from build123d import *

# Parameters (mm, degrees)
SKETCH_1_R          = 2.15
SKETCH_1_W          = 14.4
SKETCH_1_H          = 14.4
EXTRUDE_1_DEPTH     = 6
CUT_EXTRUDE_START   = -4
CUT_EXTRUDE_1_DEPTH = 4
CHAMFER_1_SIZE      = 1
SKETCH_4_W          = 5
SKETCH_4_H          = 1
CUT_EXTRUDE_2_DEPTH = 0.4


with BuildPart() as part:
    # Эскиз1 → Бобышка-Вытянуть1 (new body)
    with BuildSketch(Plane.XY):
        with BuildLine():
            Line((17.75, 16.5), (-17.75, 16.5))
            ThreePointArc((-17.75, 16.5), (-20.401650429, 15.401650429), (-21.5, 12.75))
            Line((-21.5, 12.75), (-21.5, -12.75))
            ThreePointArc((-21.5, -12.75), (-20.401650429, -15.401650429), (-17.75, -16.5))
            Line((-17.75, -16.5), (17.75, -16.5))
            ThreePointArc((17.75, -16.5), (20.401650429, -15.401650429), (21.5, -12.75))
            Line((21.5, -12.75), (21.5, 12.75))
            ThreePointArc((21.5, 12.75), (20.401650429, 15.401650429), (17.75, 16.5))
        make_face()
        with Locations((-17.75, 12.75)):
            Circle(SKETCH_1_R, mode=Mode.SUBTRACT)
        with Locations((17.75, 12.75)):
            Circle(SKETCH_1_R, mode=Mode.SUBTRACT)
        with Locations((-17.75, -12.75)):
            Circle(SKETCH_1_R, mode=Mode.SUBTRACT)
        with Locations((17.75, -12.75)):
            Circle(SKETCH_1_R, mode=Mode.SUBTRACT)
        with Locations((-9.5, 0)):
            Rectangle(SKETCH_1_W, SKETCH_1_H, mode=Mode.SUBTRACT)
        with Locations((9.5, 0)):
            Rectangle(SKETCH_1_W, SKETCH_1_H, mode=Mode.SUBTRACT)
    extrude(amount=EXTRUDE_1_DEPTH)

    # Эскиз2 → Вырез-Вытянуть1 (cut)
    with BuildSketch(Plane.XY.offset(6).offset(CUT_EXTRUDE_START)):
        with BuildLine():
            Line((-21.5, 10.25), (-20.545084972, 10.25))
            ThreePointArc((-20.545084972, 10.25), (-19.837764528, 9.634917453), (-19, 9.214466094))
            Line((-19, 9.214466094), (-19, -9.214466094))
            ThreePointArc((-19, -9.214466094), (-19.837764528, -9.634917453), (-20.545084972, -10.25))
            Line((-20.545084972, -10.25), (-21.5, -10.25))
            Line((-21.5, -10.25), (-21.5, -12.75))
            ThreePointArc((-21.5, -12.75), (-20.401650429, -15.401650429), (-17.75, -16.5))
            Line((-17.75, -16.5), (-15.25, -16.5))
            Line((-15.25, -16.5), (-15.25, -15.545084972))
            ThreePointArc((-15.25, -15.545084972), (-14.020147597, -12.361797664), (-15.879171307, -9.5))
            Line((-15.879171307, -9.5), (15.879171307, -9.5))
            ThreePointArc((15.879171307, -9.5), (14.020147597, -12.361797664), (15.25, -15.545084972))
            Line((15.25, -15.545084972), (15.25, -16.5))
            Line((15.25, -16.5), (17.75, -16.5))
            ThreePointArc((17.75, -16.5), (20.401650429, -15.401650429), (21.5, -12.75))
            Line((21.5, -12.75), (21.5, -10.25))
            Line((21.5, -10.25), (20.545084972, -10.25))
            ThreePointArc((20.545084972, -10.25), (19.837764528, -9.634917453), (19, -9.214466094))
            Line((19, -9.214466094), (19, 9.214466094))
            ThreePointArc((19, 9.214466094), (19.837764528, 9.634917453), (20.545084972, 10.25))
            Line((20.545084972, 10.25), (21.5, 10.25))
            Line((21.5, 10.25), (21.5, 12.75))
            ThreePointArc((21.5, 12.75), (20.401650429, 15.401650429), (17.75, 16.5))
            Line((17.75, 16.5), (15.25, 16.5))
            Line((15.25, 16.5), (15.25, 15.545084972))
            ThreePointArc((15.25, 15.545084972), (14.020147597, 12.361797664), (15.879171307, 9.5))
            Line((15.879171307, 9.5), (-15.879171307, 9.5))
            ThreePointArc((-15.879171307, 9.5), (-14.020147597, 12.361797664), (-15.25, 15.545084972))
            Line((-15.25, 15.545084972), (-15.25, 16.5))
            Line((-15.25, 16.5), (-17.75, 16.5))
            ThreePointArc((-17.75, 16.5), (-20.401650429, 15.401650429), (-21.5, 12.75))
            Line((-21.5, 12.75), (-21.5, 10.25))
        make_face()
    extrude(amount=CUT_EXTRUDE_1_DEPTH, mode=Mode.SUBTRACT)

    # Фаска1
    # the kernel refuses this chamfer: 1, 0.732303349 mm, written as the material it takes off along each edge
    with BuildSketch(Plane(origin=(15.879171307, 9.5, 2), x_dir=(-0.8149940779202551, 0.5794692856009827, 0), z_dir=(0, 0, 1))) as chamfer_1_piece_1:
        with BuildLine():
            Line((0.717121745, 0), (CHAMFER_1_SIZE * 0.81499407792, CHAMFER_1_SIZE * 0.579469285601))
            Line((CHAMFER_1_SIZE * 0.81499407792, CHAMFER_1_SIZE * 0.579469285601), (0, 0))
            ThreePointArc((0, 0), (0.355196947, 0.017179972), (0.717121745, 0))
        make_face()
    extrude(amount=6.571682988, mode=Mode.SUBTRACT)
    with BuildSketch(Plane(origin=(-15.879171307, 9.5, 2), x_dir=(1, 0, 0), z_dir=(0, 0, 1))) as chamfer_1_piece_2:
        with BuildLine():
            Line((CHAMFER_1_SIZE, 0), (0.584449975, 0.415550025))
            ThreePointArc((0.584449975, 0.415550025), (0.299438674, 0.191824146), (0, 0))
            Line((0, 0), (CHAMFER_1_SIZE, 0))
        make_face()
    extrude(amount=6.571682988, mode=Mode.SUBTRACT)
    with BuildSketch(Plane(origin=(15.879171307, -9.5, 2), x_dir=(-0.8149940779202558, -0.5794692856009814, 0), z_dir=(0, 0, 1))) as chamfer_1_piece_3:
        with BuildLine():
            Line((0.717121745, 0), (CHAMFER_1_SIZE * 0.81499407792, -CHAMFER_1_SIZE * 0.579469285601))
            Line((CHAMFER_1_SIZE * 0.81499407792, -CHAMFER_1_SIZE * 0.579469285601), (0, 0))
            ThreePointArc((0, 0), (0.355196947, -0.017179972), (0.717121745, 0))
        make_face()
    extrude(amount=6.571682988, mode=Mode.SUBTRACT)
    with BuildSketch(Plane(origin=(-15.879171307, -9.5, 2), x_dir=(1, 0, 0), z_dir=(0, 0, 1))) as chamfer_1_piece_4:
        with BuildLine():
            Line((CHAMFER_1_SIZE, 0), (0.584449975, -0.415550025))
            ThreePointArc((0.584449975, -0.415550025), (0.299438674, -0.191824146), (0, 0))
            Line((0, 0), (CHAMFER_1_SIZE, 0))
        make_face()
    extrude(amount=6.571682988, mode=Mode.SUBTRACT)
    with BuildSketch(Plane(origin=(21.5, -12.821682988, 6), x_dir=(0, 0, -1), z_dir=(0, 1, 0)), Plane(origin=(-21.5, 12.821682988, 6), x_dir=(0, 0, -1), z_dir=(0, -1, 0))) as chamfer_1_piece_5:
        Polygon((CHAMFER_1_SIZE, 0), (0, CHAMFER_1_SIZE), (0, 0), align=None)
    extrude(amount=25.643365976, mode=Mode.SUBTRACT)
    with BuildSketch(Plane(origin=(-17.821682988, -16.5, 6), x_dir=(0, 0, -1), z_dir=(1, 0, 0)), Plane(origin=(17.821682988, 16.5, 6), x_dir=(0, 0, -1), z_dir=(-1, 0, 0))) as chamfer_1_piece_6:
        Polygon((CHAMFER_1_SIZE, 0), (0, CHAMFER_1_SIZE), (0, 0), align=None)
    extrude(amount=35.643365976, mode=Mode.SUBTRACT)

    # Эскиз4 → Вырез-Вытянуть2 (cut)
    with BuildSketch(Plane(origin=(0, 0, 0), x_dir=(-1, 0, 0), z_dir=(0, 0, -1))):
        with Locations((9.5, -7.7)):
            Rectangle(SKETCH_4_W, SKETCH_4_H)
        with Locations((9.5, 7.7)):
            Rectangle(SKETCH_4_W, SKETCH_4_H)
        with Locations((-9.5, 7.7)):
            Rectangle(SKETCH_4_W, SKETCH_4_H)
        with Locations((-9.5, -7.7)):
            Rectangle(SKETCH_4_W, SKETCH_4_H)
    extrude(amount=-CUT_EXTRUDE_2_DEPTH, mode=Mode.SUBTRACT)


solid = part.part
For this review, take the finished solid that the model builds, in its own axes (mm). A direction names the side the tool comes from. Give positions to 0.01 mm unless a question says otherwise; leave off trailing zeros. Write each loop counter-clockwise with the first axis right and the second up, starting at its lowest first coordinate (ties: lowest second). Pieces come first, ordered by that corner, then holes. Notation, with made-up numbers: (43.25, -4) -> (54.25, -4) arc R15 ccw to (54.25, 21) -> close; hole circle Ø9 at (-15.5, 39.5). An arc over 180 degrees is marked (long way). Use CSV: the item, a comma, the result in double quotes.
Q1. To check wall thickness, follow probe 1 along Y at (x, z) = (-17.75, 1.2); probe 2 along X at (y, z) = (4.5, 4.75); probe 3 along Y at (x, z) = (0, 2.75). State the ranges of each line that lie inside material, in increasing order. Write a range as [from, to].
Conclusion:
probe 1,"[-16.5, -14.9], [-10.6, 10.6], [14.9, 16.5]"
probe 2,"[-21.5, -19], [19, 21.5]"
probe 3,"[-16.5, -9.5], [9.5, 16.5]"
Q2. Take a section at B-B, the plane z = 2.75. Write out the cut boundary in (x, y), then the cut area to 3 significant figures.
Conclusion:
outline,"(-21.5, -10.25) -> (-20.55, -10.25) arc R3.75 cw to (-19, -9.21) -> (-19, 9.21) arc R3.75 cw to (-20.55, 10.25) -> (-21.5, 10.25) -> close; (-15.29, -9.92) arc R3.75 cw to (-15.25, -15.55) -> (-15.25, -16.5) -> (15.25, -16.5) -> (15.25, -15.55) arc R3.75 cw to (15.29, -9.92) -> (14.88, -9.5) -> (-14.88, -9.5) -> close; (-15.29, 9.92) -> (-14.88, 9.5) -> (14.88, 9.5) -> (15.29, 9.92) arc R3.75 cw to (15.25, 15.55) -> (15.25, 16.5) -> (-15.25, 16.5) -> (-15.25, 15.55) arc R3.75 cw to start; (19, -9.21) arc R3.75 cw to (20.55, -10.25) -> (21.5, -10.25) -> (21.5, 10.25) -> (20.55, 10.25) arc R3.75 cw to (19, 9.21) -> close"
area,"506 mm2"
Q3. Tool access review of faces 5 (the face through (15.25, 16, 4)), 6 (the face through (21, -10.25, 4)), 7 (the face through (-15.25, 16, 4)), 8 (the face through (-19.83, -9.63, 3.97)): name each direction out of +Z, -Z, +X, -X, +Y, -Y from which nothing blocks a thin tool from reaching the whole face with its end or side.
Conclusion:
face 5,"+Z, +X, +Y"
face 6,"+Z, +X, -Y"
face 7,"+Z, -X, +Y"
face 8,"+Z, -Y"
Q4. Take a section at A-A, the plane y = -0.5. Write out the cut boundary in (x, z), then the cut area to 3 significant figures.
Conclusion:
outline,"(-21.5, 0) -> (-16.7, 0) -> (-16.7, 2) -> (-19, 2) -> (-19, 6) -> (-20.5, 6) -> (-21.5, 5) -> close; (-2.3, 0) -> (2.3, 0) -> (2.3, 2) -> (-2.3, 2) -> close; (16.7, 0) -> (21.5, 0) -> (21.5, 5) -> (20.5, 6) -> (19, 6) -> (19, 2) -> (16.7, 2) -> close"
area,"47.4 mm2"
Q5. Mouldability with a two-part tool opening along X and no side actions: class faces 1 (the face through (-0.2, -16, 5.5)), 2 (the face through (-2.3, 0, 1)), 3 (the face through (21.5, 0, 2)), 4 (the face through (19, 11, 1)) as pulls with the +X half, pulls with the -X half, needs draft (parallel to the pull), parting line crosses it, or undercut.
Conclusion:
face 1,"needs draft"
face 2,"undercut"
face 3,"pulls with the +X half"
face 4,"undercut"
Q6. For P1, Ø3, axis at x = 4, y = 6.5, coming from the +Z side; P2, Ø1.1, axis at y = 16, z = 4, coming from the +X side; P3, Ø0.5, axis at x = 21, z = 5, coming from the +Y side, all flat-tipped, find the tip position at first contact; note any pin that passes through.
Conclusion:
P1,"z = 2"
P2,"x = 15.25"
P3,"y = 10.25"
